Part model, mm, in its own coordinate system. A direction names the side the tool comes from. Round coordinates to 2 decimals unless told otherwise and drop trailing zeros. Loops run counter-clockwise (first coordinate to the right, second up) from the corner with the lowest first, then second, coordinate; pieces in that order, holes last. Notation, with made-up numbers: (16.25, 53) -> (50.25, 53) arc R17 ccw to (50.25, 84) -> close; hole circle Ø7 at (37, 12.25). An arc over 180 degrees is marked (long way). Answer as a JSON object with one key per item and string values. Group by question number.
from build123d import *

# Parameters (mm, degrees)
F0_W     = 25.4
F0_H     = 25.4
F1_DEPTH = 63.5


with BuildPart() as f1:
    # F0 (on Top) → F1 (new body, symmetric)
    with BuildSketch(Plane.XY):
        with BuildLine():
            Line((-12.7, 58.4446051985), (0, 58.4446051985))
            Line((0, 58.4446051985), (12.7, 58.4446051985))
            ThreePointArc((12.7, 58.4446051985), (9.1177237853, 68.4465950708), (0, 73.8999992609))
            ThreePointArc((0, 73.8999992609), (-9.1177237853, 68.4465950708), (-12.7, 58.4446051985))
        make_face()
        Polygon((12.7, 58.4446051985), (0, 58.4446051985), (-12.7, 58.4446051985), (-12.7, 33.0446051985), (-38.1, 33.0446051985), (-38.1, 7.6446051985), (-12.7, 7.6446051985), (-12.7, -16.1055155754), (-12.7, -41.5055155754), (-12.7, -49.8682335019), (12.7, -49.8682335019), (12.7, -41.5055155754), (12.7, -16.1055155754), (12.7, 8.3362860605), (38.1, 8.3362860605), (38.1, 33.0446051985), (12.7, 33.0446051985), (12.7, 45.7446051985), align=None)
        with BuildLine():
            ThreePointArc((38.1, 33.0446051985), (20.1394877579, 40.4840929564), (12.7, 58.4446051985))
            Line((12.7, 58.4446051985), (12.7, 45.7446051985))
            Line((12.7, 45.7446051985), (12.7, 33.0446051985))
            Line((12.7, 33.0446051985), (38.1, 33.0446051985))
        make_face()
        with BuildLine():
            Line((-12.7, 33.0446051985), (-12.7, 58.4446051985))
            ThreePointArc((-12.7, 58.4446051985), (-20.1394877579, 40.4840929564), (-38.1, 33.0446051985))
            Line((-38.1, 33.0446051985), (-12.7, 33.0446051985))
        make_face()
        with BuildLine():
            ThreePointArc((53.8339801133, 20.6904456295), (48.1022920981, 29.5869981283), (38.1, 33.0446051985))
            Line((38.1, 33.0446051985), (38.1, 8.3362860605))
            ThreePointArc((38.1, 8.3362860605), (48.1022920981, 11.7938931307), (53.8339801133, 20.6904456295))
        make_face()
        with BuildLine():
            Line((-38.1, 7.6446051985), (-38.1, 33.0446051985))
            ThreePointArc((-38.1, 33.0446051985), (-48.1779241379, 30.1618280155), (-55.2068687975, 22.3856531084))
            ThreePointArc((-55.2068687975, 22.3856531084), (-49.3909637934, 11.8382480748), (-38.1, 7.6446051985))
        make_face()
        with BuildLine():
            ThreePointArc((29.4168628752, -3.037011018), (30.9454777105, 4.7972348951), (38.1, 8.3362860605))
            Line((38.1, 8.3362860605), (12.7, 8.3362860605))
            Line((12.7, 8.3362860605), (12.7, -16.1055155754))
            Line((12.7, -16.1055155754), (38.1, -16.1055155754))
            ThreePointArc((38.1, -16.1055155754), (37.8112363374, -15.9115868292), (37.5258770827, -15.7126825627))
            ThreePointArc((37.5258770827, -15.7126825627), (32.2384158105, -10.1636052268), (29.4168628752, -3.037011018))
        make_face()
        with BuildLine():
            Line((-12.7, 7.6446051985), (-38.1, 7.6446051985))
            ThreePointArc((-38.1, 7.6446051985), (-29.6939751713, 4.5068420563), (-25.4, -3.3715199679))
            ThreePointArc((-25.4, -3.3715199679), (-29.107716584, -12.3737471543), (-38.1, -16.1055155754))
            Line((-38.1, -16.1055155754), (-12.7, -16.1055155754))
            Line((-12.7, -16.1055155754), (-12.7, 7.6446051985))
        make_face()
        with BuildLine():
            ThreePointArc((60.5236142874, -26.4526233077), (50.436987874, -18.0585790132), (37.5258770827, -15.7126825627))
            ThreePointArc((37.5258770827, -15.7126825627), (37.8112363374, -15.9115868292), (38.1, -16.1055155754))
            Line((38.1, -16.1055155754), (38.1, -41.5055155754))
            Line((38.1, -41.5055155754), (12.7, -41.5055155754))
            Line((12.7, -41.5055155754), (12.7, -49.8682335019))
            Line((12.7, -49.8682335019), (-12.7, -49.8682335019))
            Line((-12.7, -49.8682335019), (-12.7, -41.5055155754))
            Line((-12.7, -41.5055155754), (-38.1, -41.5055155754))
            ThreePointArc((-38.1, -41.5055155754), (-37.9658127793, -56.6748011531), (-28.7389459174, -68.7159871021))
            ThreePointArc((-28.7389459174, -68.7159871021), (4.3955551034, -83.6780580167), (38.4478494525, -70.9422826767))
            ThreePointArc((38.4478494525, -70.9422826767), (63.1143336959, -55.4599639488), (60.5236142874, -26.4526233077))
        make_face()
        with Locations((-25.4, -28.8055155754)):
            Rectangle(F0_W, F0_H)
        with BuildLine():
            Line((-38.1, -41.5055155754), (-38.1, -16.1055155754))
            ThreePointArc((-38.1, -16.1055155754), (-50.8550498174, -19.5062062845), (-60.2240860462, -28.8055155754))
            ThreePointArc((-60.2240860462, -28.8055155754), (-50.8550498174, -38.1048248663), (-38.1, -41.5055155754))
        make_face()
        with BuildLine():
            ThreePointArc((-28.7389459174, -68.7159871021), (-37.9658127793, -56.6748011531), (-38.1, -41.5055155754))
            ThreePointArc((-38.1, -41.5055155754), (-50.8550498174, -38.1048248663), (-60.2240860462, -28.8055155754))
            ThreePointArc((-60.2240860462, -28.8055155754), (-60.9967813298, -61.7895486407), (-28.7389459174, -68.7159871021))
        make_face()
    extrude(amount=F1_DEPTH, both=True)


solid = f1.part
Item 1: Band-saw the part on D-D, the plane y = -5.5. List the corners of the cut face in (x, z).
Item 2: Drop flat-ended pins along their axis: pin 1 Ø20.5 at (x, z) = (27, 13) entering from +Y; pin 2 Ø20.5 at (y, z) = (-28.5, -16.5) entering from -X; pin 3 Ø3 at (y, z) = (40.5, -8.5) entering from -X. Give the stop position or say it passes through.
Item 3: Band-saw the part on C-C, the plane y = -32. List the corners of the cut face in (x, z), plus the area to 3 significant figures.
Item 4: Drill centre lines: line 1 (Y direction, x = 31, z = -42.5); line 2 (Y direction, x = 20, z = -34.5); line 3 (Y direction, x = 40.5, z = 34). Where is each one in solid material? Low to high.
Item 5: Band-saw the part on A-A, the plane x = 16. List the corners of the cut face in (y, z).
Item 6: Which spindle directions (+Z, -Z, +X, -X, +Y, -Y) get a long thin tool onto all of the face, cutting with end or side? Do faces 1 (the face through (-19.943, 40.683, 0.889)), 2 (the face through (20.338, 40.288, 0.889)), 3 (the face through (26, -41.506, 1)), 4 (the face through (47.98, 11.7, 0.89)), 5 (the face through (-49.52, 11.95, 0.89)). Say none if no direction does.
Item 7: Two-plate mould, pull along Y, no slides. Class faces 6 (the face through (-48.05, 30.24, 0.89)), 7 (the face through (-1, -21, -63.5)), 8 (the face through (50.61, -18.14, 0.89)): pulls with the +Y half, pulls with the -Y half, needs draft (parallel to the pull), parting line crosses it, or undercut.
Item 8: Band-saw the part on B-B, the plane z = 10. List the corners of the cut face in (x, y) (3 decimals), plus the area to 3 significant figures.
Entries:
{
 "1": {"outline": "(-25.57, -63.5) -> (30.04, -63.5) -> (30.04, 63.5) -> (-25.57, 63.5) -> close"},
 "2": {"pin 1": "y = 44.68", "pin 2": "x = -65.59", "pin 3": "x = -21.76"},
 "3": {"outline": "(-62.59, -63.5) -> (12.7, -63.5) -> (12.7, 63.5) -> (-62.59, 63.5) -> close; (38.1, -63.5) -> (63.73, -63.5) -> (63.73, 63.5) -> (38.1, 63.5) -> close", "area": "12,800 mm²"},
 "4": {"line 1": "-76.61 to -41.51, -16.11 to -7.93, 4.87 to 34.06", "line 2": "-81.6 to -41.51, -16.11 to 40.62", "line 3": "-70.84 to -15.65, 8.52 to 32.87"},
 "5": {"outline": "(-82.64, -63.5) -> (-41.51, -63.5) -> (-41.51, 63.5) -> (-82.64, 63.5) -> close; (-16.11, -63.5) -> (45.92, -63.5) -> (45.92, 63.5) -> (-16.11, 63.5) -> close"},
 "6": {"face 1": "+Z, -Z, -X, +Y", "face 2": "+Z, -Z, +X, +Y", "face 3": "+Z, -Z", "face 4": "+Z, -Z, +X", "face 5": "+Z, -Z, -X"},
 "7": {"face 6": "pulls with the +Y half", "face 7": "needs draft", "face 8": "undercut"},
 "8": {"outline": "(-60.224, -28.806) arc R25.874 ccw to (-28.739, -68.716) arc R47.694 ccw to (38.448, -70.942) arc R27.873 ccw to (60.524, -26.453) arc R25.797 ccw to (37.526, -15.713) arc R20.069 cw to (29.417, -3.037) arc R9.001 cw to (38.1, 8.336) arc R16.196 ccw to (53.834, 20.69) arc R16.196 ccw to (38.1, 33.045) arc R25.4 cw to (12.7, 58.445) arc R15.754 ccw to (0, 73.9) arc R15.754 ccw to (-12.7, 58.445) arc R25.4 cw to (-38.1, 33.045) arc R19.057 ccw to (-55.207, 22.386) arc R17.297 ccw to (-38.1, 7.645) arc R12.829 cw to (-25.4, -3.372) arc R12.7 cw to (-38.1, -16.106) arc R25.621 ccw to start; hole (12.7, -41.506) -> (38.1, -41.506) -> (38.1, -16.106) -> (12.7, -16.106) -> close", "area": "11,700 mm²"}
}
